Part print with two shaded views. Sizes in mm from the minimum x, y, z corner. Give positions to 0.01 mm unless a question says otherwise; leave off trailing zeros. Write each loop counter-clockwise with the first axis right and the second up, starting at its lowest first coordinate (ties: lowest second). Pieces come first, ordered by that corner, then holes. Notation, with made-up numbers: M -11,53 L 36,53 A20 ccw 36,78 Z; hole C 6.5,67.25 d5. An arc over 180 degrees is marked long. Return JSON: item names as keys, results as strings. Group by question number.
Q1. Band-saw the part on A-A, the plane z = 113. Give the cut face in (x, y) (1 decimal).
Q2. Pull direction Y, two halves, no side cores. Call the marked faces 1 and 2: +Y half, -Y half, draft (parallel to the pull), parting line (faces both ways), or undercut.
Q3. Flat gauge pins, fed straight in: pin 1 Ø5 at (y, z) = (5.5, 116) entering from +X (1 decimal); pin 2 Ø6 at (x, z) = (21, 43) entering from -Y; pin 3 Ø3 at (y, z) = (3.5, 26.5) entering from -X (1 decimal); pin 4 Ø3 at (x, y) = (17, 27.5) entering from +Z. Where does each tip first touch, or does it go through?
Q4. Band-saw the part on C-C, the plane z = 18. Give the cut face in (x, y) (1 decimal).
Q5. Band-saw the part on B-B, the plane x = 10. Give the cut face in (y, z) (1 decimal).
Q6. Wall check: probe 1 along Y at (x, z) = (17.5, 44); probe 2 along Y at (x, z) = (12.5, 9) (1 decimal). Give the ranges that are in metal, low to high.
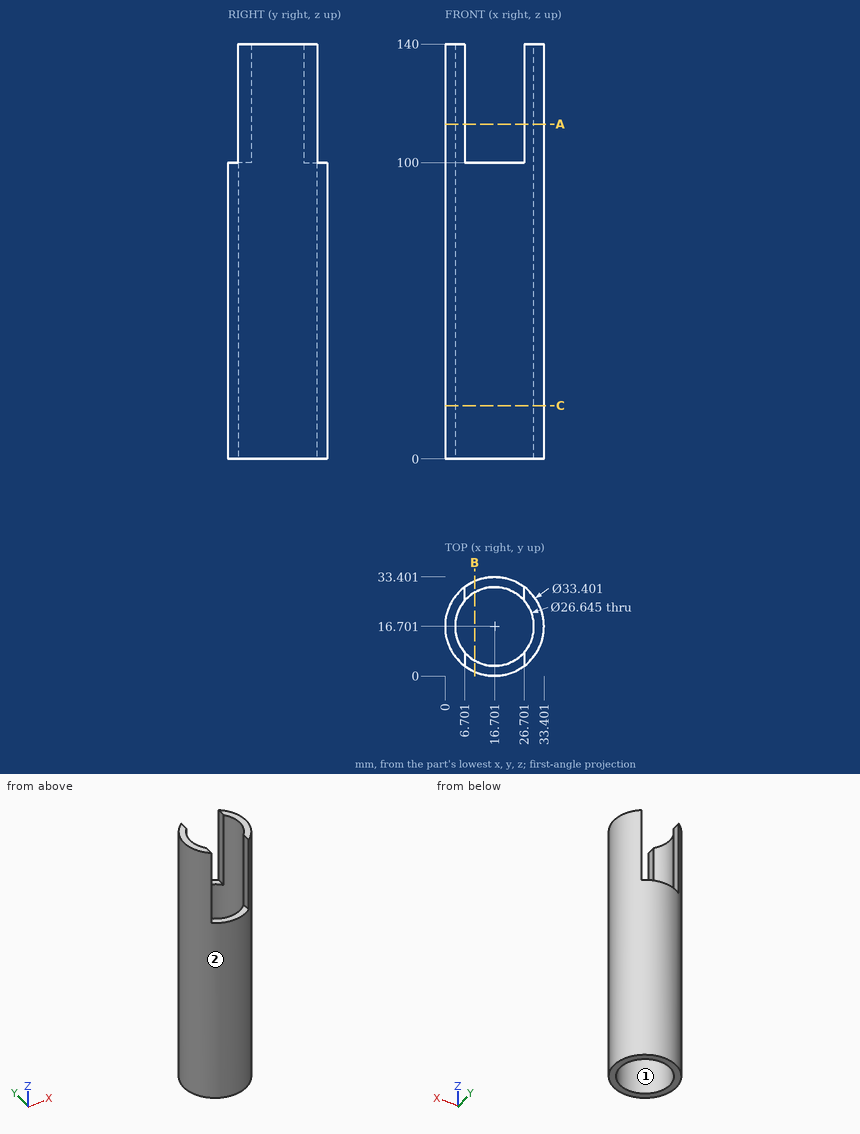
From the geometry:
{
 "1": {"outline": "M 6.7,3.3 L 6.7,7.9 A13.3 cw 6.7,25.5 L 6.7,30.1 A16.7 ccw Z; M 26.7,3.3 A16.7 ccw 26.7,30.1 L 26.7,25.5 A13.3 cw 26.7,7.9 Z"},
 "2": {"face 1": "undercut", "face 2": "parting line"},
 "3": {"pin 1": "stops at x = 31", "pin 2": "stops at y = 0.05", "pin 3": "stops at x = 4.8", "pin 4": "passes through"},
 "4": {"outline": "C 16.7,16.7 d33.4; hole C 16.7,16.7 d26.6"},
 "5": {"outline": "M 1.4,0 L 5.2,0 L 5.2,100 L 1.4,100 Z; M 28.2,0 L 32,0 L 32,100 L 28.2,100 Z"},
 "6": {"probe 1": "y = 0.02 to 3.4, 30 to 33.38", "probe 2": "y = 0.5 to 4.1, 29.3 to 32.9"}
}
